Could you check a few things on this drawing? It's one solid part, dimensions in mm from its lowest x, y, z. Coordinates: 2 decimals unless noted, no trailing zeros.
1) Will these pins go through, and if not, where does the flat tip stop? P1, Ø2, axis at y = 3.5, z = 0.5, coming from the -X side; P2, Ø1.5, axis at x = 1.5, z = 4.5, coming from the +Y side.
2) Thinking about a two-plate mould opening in Z: for the marked faces 1, 2, 3 and 4, which applies, released by +Z, released by -Z, zero draft, split by the parting line, or undercut?
3) If I drill on line 1 along Y through (x, z) = (2.6, 2.75) (1 decimal); line 2 along Y through (x, z) = (3.7, 2.1) (1 decimal); line 3 along Z through (x, y) = (3.45, 3.75), over which ranges is the centre line in solid material (lowest first)?
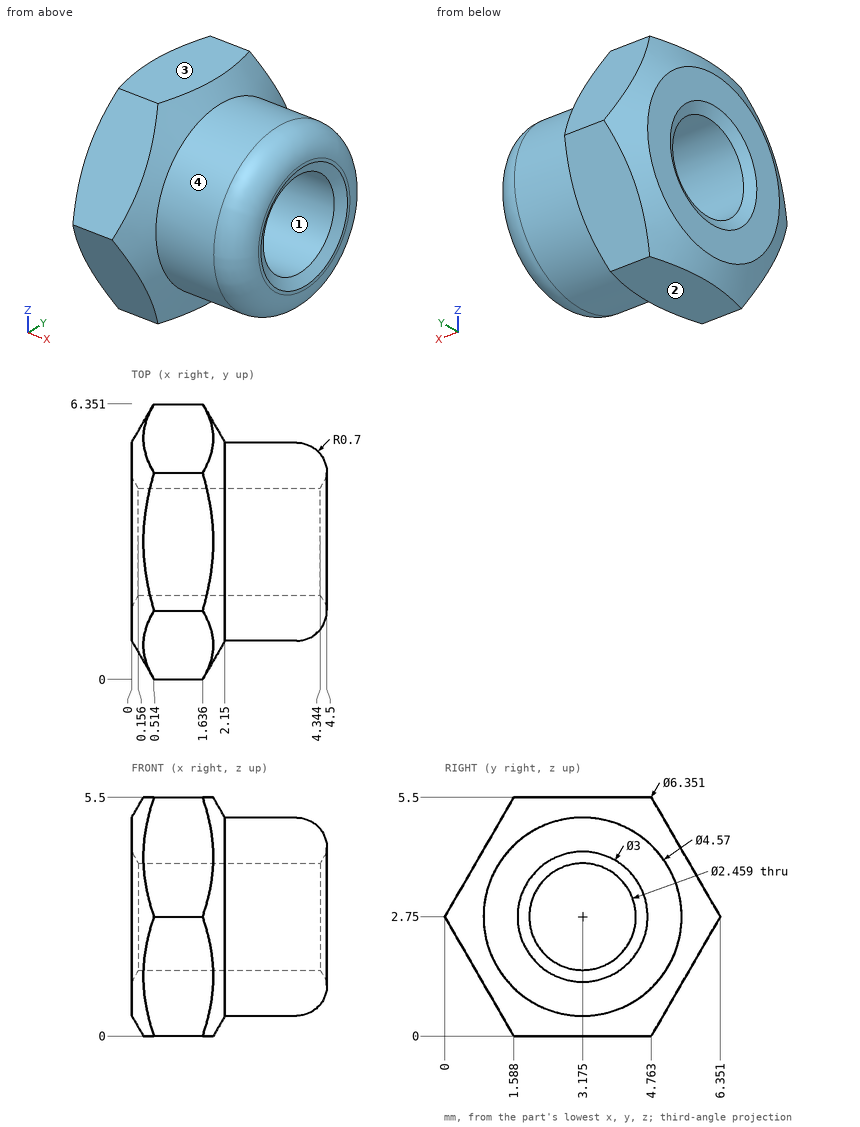
Filled in:
1. P1: stops at x = 0
1. P2: stops at y = 5.77
2. face 1: undercut
2. face 2: released by -Z
2. face 3: released by +Z
2. face 4: split by the parting line
3. line 1: y = 0.9 to 1.9, 4.4 to 5.5
3. line 2: y = 1 to 2.1, 4.2 to 5.4
3. line 3: z = 0.54 to 1.66, 3.84 to 4.96
